Can you work these out from the drawing? Everything is in mm from the part's minimum corner. A direction names the side the tool comes from. Coordinates: 2 decimals unless noted, no trailing zeros. Write each loop counter-clockwise with the first axis right and the second up, starting at its lowest first coordinate (ties: lowest second). Pieces come first, ordered by that corner, then holes. Notation, with made-up numbers: M 80,77 L 100,77 A27 cw 100,95 Z; hole C -37.75,-21.5 d5. An arc over 180 degrees is marked long. Write item = value, one per line.
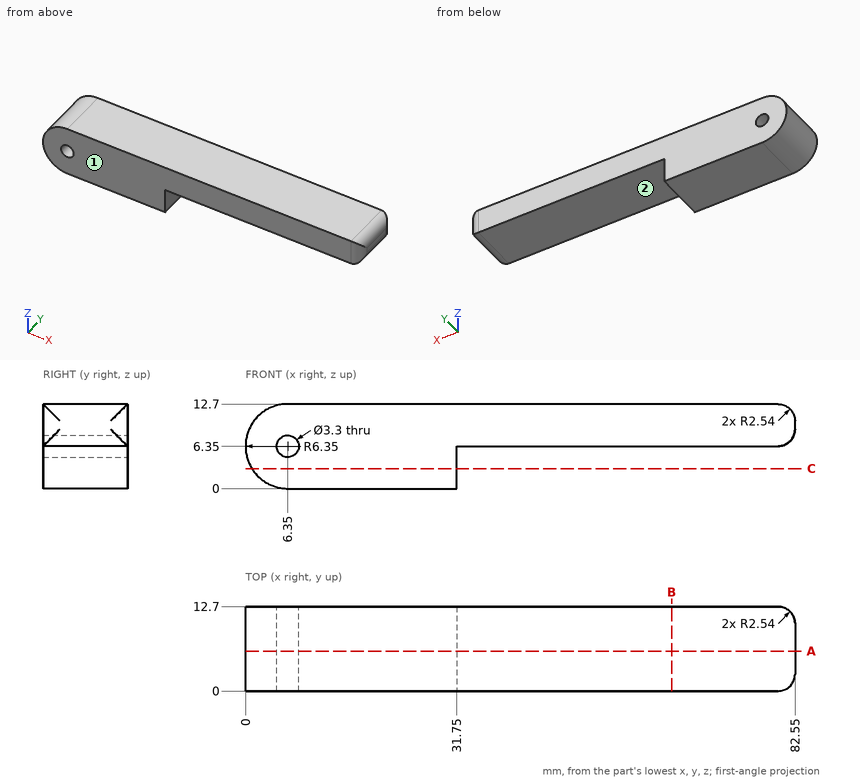
Item 1: I'm going to push flat-ended pins straight in: P1, Ø1.9, axis at y = 6, z = 2, coming from the +X side; P2, Ø6, axis at y = 9, z = 10.5, coming from the -X side (3 decimals); P3, Ø3, axis at x = 61.5, y = 5.5, coming from the -Z side. Where does each tip first touch, or does it pass through?
Numbers:
P1 = 31.75
P2 = 0.105
P3 = 6.35
Item 2: Imagine slicing it at B-B (x = 64). Write out the boundary of the cut face in (y, z).
Numbers:
outline = M 0,6.35 L 12.7,6.35 L 12.7,12.7 L 0,12.7 Z
Item 3: If I drill on line 1 along Z through (x, y) = (6.35, 6.25); line 2 along Z through (x, y) = (77.5, 9.75), over which ranges is the centre line in solid material (lowest first)?
Numbers:
line_1 = 0 to 4.7, 8 to 12.7
line_2 = 6.35 to 12.7
Item 4: Imagine slicing it at A-A (y = 6). Write out the boundary of the cut face in (x, z).
Numbers:
outline = M 6.35,0 L 31.75,0 L 31.75,6.35 L 80.01,6.35 A2.54 ccw 82.55,8.89 L 82.55,10.16 A2.54 ccw 80.01,12.7 L 6.35,12.7 A6.35 ccw Z; hole C 6.35,6.35 d3.3
Item 5: For the marked faces 1 and 2, which set-ups out of +Z, -Z, +X, -X, +Y, -Y let a thin tool reach every point of the face, with its end or its side?
Numbers:
face_1 = +Z, -Z, +X, -X, -Y
face_2 = -Z, +X, +Y, -Y
Item 6: Imagine slicing it at C-C (z = 3). Write out the boundary of the cut face in (x, y).
Numbers:
outline = M 0.96,0 L 31.75,0 L 31.75,12.7 L 0.96,12.7 Z
